The listing builds one solid part. Answer for the finished solid, in the listing's coordinates (mm). A direction names the side the tool comes from. Give positions to 0.01 mm unless a question says otherwise; leave off trailing zeros. Loops run counter-clockwise (first coordinate to the right, second up) from the corner with the lowest first, then second, coordinate; pieces in that order, holes last.
Item 1: A tool of negligible diameter and unlimited length cuts with its end or side. For faces 4 (the face through (30.033, 21.322, 2.027)), 5 (the face through (-9.41, -0.6, 14.43)), 6 (the face through (-9, 47, 15)), 7 (the face through (4, 0, -1)), from which of +Z, -Z, +X, -X, +Y, -Y can it reach the whole face along a straight path? Write none if from no direction.
Item 2: The mould has two halves that part along Y. Classify faces 1 (the face through (-21.981, -5, 2)), 2 (the face through (5, 50, 0)), 3 (the face through (3, 42, -1)): pulls with the +Y half, pulls with the -Y half, needs draft (parallel to the pull), parting line crosses it, or undercut.
Item 3: Consider line 1 along Y through (x, z) = (24, 3.5); line 2 along X through (y, z) = (36.5, -6); line 3 along X through (y, z) = (46, 8). Determine where each line is inside the solid, lowest interval first.
Item 4: Section A-A, the plane x = -8 is taken. Give the vertices of the cut face in (y, z).
Item 5: Each of these flat-tipped pins is pushed along its axis until it touches: pin 1 Ø1.5 at (y, z) = (21.5, -11) entering from -X; pin 2 Ø8 at (x, y) = (14.5, 3) entering from -Z. Where does it stop, or does it pass through?
Item 6: Section C-C, the plane y = 28.5 is taken. Give the vertices of the cut face in (x, z).
Item 7: Section B-B, the plane z = -4.5 is taken. Give the vertices of the cut face in (x, y), and give its area (3 significant figures).
Item 8: Section D-D, the plane x = -14.5 is taken. Give the vertices of the cut face in (y, z).
Autodesk Inventor part; units mm, degrees
ref_plane "YZ Plane" through (0, 0, 0) normal (1, 0, 0) x (0, 1, 0)
ref_plane "XZ Plane" through (0, 0, 0) normal (0, 1, 0) x (-1, 0, 0)
ref_plane "XY Plane" through (0, 0, 0) normal (0, 0, 1) x (1, 0, 0)
sketch "Skizze1" plane through (0, 0, 0) normal (0, 0, 1) x (1, 0, 0)
  line L0 (9, 36) -> (9, 6) construction
  line L1 (-9, 36) -> (9, 36) construction
  line L2 (-9, 6) -> (-9, 36) construction
  line L3 (-9, 6) -> (9, 6) construction
  line L4 (9, 36) -> (9, 6) construction
  line L5 (-9, 42) -> (9, 42) construction
  line L6 (9, 6) -> (9, 0) construction
  line L7 (-9, 42) -> (-31, 42) construction
  line L8 (2.1623, -5) -> (-7.3221, -5) construction
  line L9 (-9, 0) -> (9, 0) construction
  line L10 (2.1623, 6.8548) -> (2.1623, -5) construction
  line L11 (4.0374, -5) -> (4.0374, 6.8548) construction
  line L12 (4.0374, -5) -> (2.1623, -5) construction
  line L13 (9, 42) -> (9, 36) construction
  line L14 (32.5442, 50) -> (-21.2, 50) construction
  line L15 (-22.4813, -15) -> (-22.4813, 53) construction
  arc A0 (-22.4813, 53) -> (-24.4813, 55) centre (-24.4813, 53) ccw construction
  arc A1 (-24.6813, -15) -> (-22.6813, -13) centre (-24.6813, -13) ccw construction
  line L16 (-22.6813, -13) -> (-22.6813, -12) construction
  line L17 (-24.4813, -13) -> (-47, -13) construction
  line L18 (-24.4813, 53) -> (-24.4813, -13) construction
  line L19 (-47, 53) -> (-24.4813, 53) construction
  line L20 (-47, -13) -> (-47, 53) construction
  line L21 (-9, 6) -> (-9, 0) construction
  line L22 (-8.7, -6) -> (-8.7, -4) construction
  line L23 (-8.7, -6) -> (-8.7, -4) construction
  line L24 (-8.7, -4) -> (-7.7, -4) construction
  line L25 (-7.7, -4) -> (-7.7, -6) construction
  line L26 (-7.7, -6) -> (-4.7, -6) construction
  line L27 (-4.7, 1) -> (-4.7, -6) construction
  line L28 (-4.7, 1) -> (-9.7, 1) construction
  line L29 (-9.7, 1) -> (-9.7, -6) construction
  line L30 (-9.7, -6) -> (-8.7, -6) construction
  line L31 (-9, 0.5858) -> (-9, 7.4142) construction
  line L32 (-31, 0) -> (-9, 0) construction
  line L33 (-21.2, 52) -> (-21.2, 50) construction
  line L34 (-21.2, -10) -> (32.5442, -10) construction
  line L35 (-21.2, -10) -> (-21.2, -12) construction
  line L36 (32.2, 50) -> (32.2, 35.4011) construction
  line L37 (32.2, 4.5989) -> (32.2, -10) construction
  line L38 (-21.9813, -10) -> (32.2, -10)
  line L39 (32.2, -10) -> (32.2, 50)
  line L40 (32.2, 50) -> (-21.9813, 50)
  line L41 (-21.9813, 42) -> (29.0187, 42)
  line L42 (29.0187, 42) -> (29.0187, 0)
  line L43 (29.0187, 0) -> (-21.9813, 0)
  line L44 (-21.9813, -10) -> (-21.9813, 0)
  line L45 (-21.9813, 42) -> (-21.9813, 50)
  point P0 (0, 0)
extrude "Extrusion1" add sketch "Skizze1" along normal mid plane 30
sketch "Skizze2" plane through (-21.9813, 50, 15) normal (0, 1, 0) x (1, 0, 0)
  circle A0 centre (33.5439, 8.6575) radius 2.15 construction
  circle A1 centre (12.1205, 3.0946) radius 2.15 construction
  arc A2 (-10.3687, -0.3954) -> (-6.0687, -0.3954) centre (-8.2187, -0.3954) ccw construction
  line L0 (-10.3687, -0.3954) -> (-10.3687, 4.6046) construction
  arc A3 (-6.0687, 4.6046) -> (-10.3687, 4.6046) centre (-8.2187, 4.6046) ccw construction
  line L1 (-6.0687, 4.6046) -> (-6.0687, -0.3954) construction
  line L2 (-6.0687, 21.1993) -> (-6.0687, 16.1993) construction
  arc A4 (-10.3687, 16.1993) -> (-6.0687, 16.1993) centre (-8.2187, 16.1993) ccw construction
  line L3 (-10.3687, 16.1993) -> (-10.3687, 21.1993) construction
  arc A5 (-6.0687, 21.1993) -> (-10.3687, 21.1993) centre (-8.2187, 21.1993) ccw construction
  line L4 (58.3, 29.6207) -> (63.3, 29.6207) construction
  line L5 (58.3, 29.6207) -> (58.3, 23.282) construction
  line L6 (58.3, 23.282) -> (57.1813, 23.282) construction
  line L7 (57.1813, 23.282) -> (57.1813, 29.0056) construction
  arc A6 (-9.2981, 25.6207) -> (57.1813, 29.0056) centre (18.9366, 125.6108) ccw construction
  line L8 (-18.2187, 25.6207) -> (-9.2981, 25.6207) construction
  line L9 (-18.2187, -4.3793) -> (-18.2187, 25.6207) construction
  line L10 (-2.7, -4.3793) -> (-18.2187, -4.3793) construction
  arc A7 (-0.7916, -2.3814) -> (-2.7, -4.3793) centre (-0.7, -4.3793) ccw construction
  arc A8 (-0.7916, -2.3814) -> (63.3, 22.1907) centre (-5.7872, 106.5198) ccw construction
  line L11 (63.3, 29.6207) -> (63.3, 22.1907) construction
  arc A9 (-0.7, -4.3793) -> (62.5308, 19.0147) centre (-5.7872, 106.5198) ccw construction
  arc A10 (-0.7, 25.6207) -> (57.1813, 31.16) centre (18.9366, 125.6108) ccw construction
  arc A11 (-0.7, 25.6207) -> (57.1813, 31.16) centre (18.9366, 125.6108) ccw construction
  line L12 (51, 0) -> (0, 0) construction
  line L13 (54.1813, 0) -> (54.1813, 30) construction
  arc A12 (25.5, 0) -> (54.1813, 13.0946) centre (-5.8671, 106.662) ccw
  line L14 (0, 0) -> (0, 30) construction
  arc A13 (0, 25.4858) -> (54.1813, 30) centre (18.9366, 125.6108) ccw
  line L15 (54.1813, 0) -> (25.5, 0)
  line L16 (54.1813, 13.0946) -> (54.1813, 0)
  line L17 (0, 25.9057) -> (0, 30)
  line L18 (0, 30) -> (51, 30)
  line L19 (0, 30) -> (54.1813, 30)
  line L20 (0, 25.9057) -> (0, 25.4858)
  point P0 (21.9813, 15)
extrude "Extrusion2" cut sketch "Skizze2" against normal through all
fillet "Rundung1" radius 2 5 edges at (16.6181, 0, 10.237) (-9.2313, 0, 15) (-9.2313, 42, 15) (16.6181, 42, 10.237) (29.0187, 21, 3.8723)
properties part number "Stiff_motor"
Worked answers:
1. face 4: +Z
1. face 5: +Z, +X, -X
1. face 6: +Z, +X, -X, +Y, -Y
1. face 7: +Z, -Z, -X
2. face 1: needs draft
2. face 2: pulls with the +Y half
2. face 3: undercut
3. line 1: y = -10 to 0, 42 to 50
3. line 2: x = 29.02 to 32.2
3. line 3: x = -21.98 to 21.43
4. outline: (-10, -8.83) - (0, -8.83) - (0, 13) arc R2 ccw to (-2, 15) - (-10, 15) - close; (42, -8.83) - (50, -8.83) - (50, 15) - (44, 15) arc R2 ccw to (42, 13) - close
5. pin 1: stops at x = 29.02
5. pin 2: stops at z = -10.73
6. outline: (29.02, -13.89) arc R101.9 cw to (32.2, -15) - (32.2, 1.91) arc R111.18 ccw to (32.1, 1.97) arc R2 ccw to (29.02, 0.29) - close
7. outline: (-21.98, -10) - (32.2, -10) - (32.2, 50) - (-21.98, 50) - (-21.98, 42) - (29.02, 42) - (29.02, 0) - (-21.98, 0) - close
7. area: 1,110 mm2
8. outline: (-10, -9.36) - (0, -9.36) - (0, 13) arc R2 ccw to (-2, 15) - (-10, 15) - close; (42, -9.36) - (50, -9.36) - (50, 15) - (44, 15) arc R2 ccw to (42, 13) - close
